```python
from build123d import *

# Parameters (mm, degrees)
SKETCH1_R               = 125
BOSS_EXTRUDE1_DEPTH     = 300
SKETCH2_W               = 100
SKETCH2_H               = 250
CUT_EXTRUDE1_DEPTH      = 200
SKETCH4_R               = 50
CUT_EXTRUDE3_DEPTH      = 60
SKETCH7_R               = 25
CUT_EXTRUDE6_DEPTH      = 176
CUT_EXTRUDE6_DEPTH_BACK = 76
FILLET2_R               = 10
SKETCH8_R               = 45
SKETCH8_R_2             = 25
CUT_EXTRUDE7_DEPTH      = 10
SKETCH10_R              = 45
SKETCH10_R_2            = 25
CUT_EXTRUDE8_DEPTH      = 10


with BuildPart() as part:
    # Sketch1 → Boss-Extrude1 (new body)
    with BuildSketch(Plane(origin=(0, 0, 0), x_dir=(1, 0, 0), z_dir=(0, 1, 0))):
        Circle(SKETCH1_R)
    extrude(amount=BOSS_EXTRUDE1_DEPTH)

    # Sketch2 → Cut-Extrude1 (cut)
    with BuildSketch(Plane(origin=(0, 300, 0), x_dir=(1, 0, 0), z_dir=(0, 1, 0))):
        Rectangle(SKETCH2_W, SKETCH2_H)
    extrude(amount=-CUT_EXTRUDE1_DEPTH, mode=Mode.SUBTRACT)

    # Sketch4 → Cut-Extrude3 (cut)
    with BuildSketch(Plane.XZ):
        Circle(SKETCH4_R)
    extrude(amount=-CUT_EXTRUDE3_DEPTH, mode=Mode.SUBTRACT)

    # Sketch7 → Cut-Extrude6 (cut, two sides)
    with BuildSketch(Plane(origin=(-50, 0, 0), x_dir=(0, 0, -1), z_dir=(1, 0, 0))) as cut_extrude6_sk:
        with BuildLine():
            Line((-87.177978871, 300), (-114.564392374, 300))
            Line((-114.564392374, 300), (-114.564392374, 235))
            ThreePointArc((-114.564392374, 235), (-105.977573518, 269.651471545), (-87.177978871, 300))
        make_face()
        with BuildLine():
            ThreePointArc((87.177978871, 300), (105.977573518, 269.651471545), (114.564392374, 235))
            Line((114.564392374, 235), (114.564392374, 300))
            Line((114.564392374, 300), (87.177978871, 300))
        make_face()
        with Locations((0, 225)):
            Circle(SKETCH7_R)
    extrude(amount=CUT_EXTRUDE6_DEPTH, mode=Mode.SUBTRACT)
    extrude(cut_extrude6_sk.sketch, amount=-CUT_EXTRUDE6_DEPTH_BACK, mode=Mode.SUBTRACT)

    # Fillet2
    fillet2_edges = [part.edges().sort_by_distance(p)[0] for p in [
        (115.807589436, 300, 47.048934409),
        (-125, 300, 0),
    ]]
    fillet(fillet2_edges, radius=FILLET2_R)

    # Sketch8 → Cut-Extrude7 (cut)
    with BuildSketch(Plane(origin=(-125, 0, 0), x_dir=(0, 0, -1), z_dir=(1, 0, 0))):
        with Locations((0, 225)):
            Circle(SKETCH8_R)
        with Locations((0, 225)):
            Circle(SKETCH8_R_2, mode=Mode.SUBTRACT)
    extrude(amount=CUT_EXTRUDE7_DEPTH, mode=Mode.SUBTRACT)

    # Sketch10 → Cut-Extrude8 (cut)
    with BuildSketch(Plane.ZY.offset(-125)):
        with Locations((0, 225)):
            Circle(SKETCH10_R)
        with Locations((0, 225)):
            Circle(SKETCH10_R_2, mode=Mode.SUBTRACT)
    extrude(amount=CUT_EXTRUDE8_DEPTH, mode=Mode.SUBTRACT)


solid = part.part
```
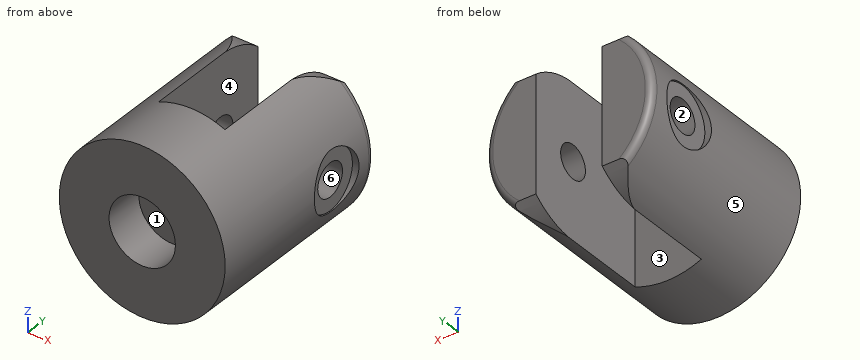
The model under review builds one solid part; all positions refer to its coordinate system, in mm. Face numbers are marked on the shaded views. A direction names the side the tool comes from. Round coordinates to 2 decimals unless told otherwise and drop trailing zeros. Order: outer loops, then holes, each group sorted by start corner. A loop starts at its lowest first (then second) coordinate and runs counter-clockwise, first axis right, second up.
(1) Take a section at C-C, the plane x = 0. State the section outline as (y, z) points.
Working result:
outline: (0, -125) - (100, -125) - (100, 125) - (0, 125) - (0, 50) - (60, 50) - (60, -50) - (0, -50) - close
(2) Tool access review of the marked faces 1, 2 and 3: name each direction out of +Z, -Z, +X, -X, +Y, -Y from which nothing blocks a thin tool from reaching the whole face with its end or side.
Working result:
face 1: -Y
face 2: +X, -X
face 3: +Z, -Z, +Y
(3) For P1, Ø5, axis at y = 58, z = -43.5, coming from the +X side; P2, Ø6, axis at y = 199.5, z = 21.5, coming from the -X side; P3, Ø3, axis at y = 137.5, z = -57, coming from the -X side, all flat-tipped, find the tip position at first contact; note any pin that passes through.
Working result:
P1: stops at x = 118.08
P2: stops at x = -115
P3: stops at x = -112
(4) Mouldability with a two-part tool opening along X and no side actions: class the marked faces 4, 5 and 6 as released by +X, released by -X, zero draft, split by the parting line, or undercut.
Working result:
face 4: undercut
face 5: split by the parting line
face 6: zero draft
(5) Take a section at A-A, the plane z = 0. Count the separate pieces of the cut face and the enclosed holes in it, plus the area to 3 significant figures.
Working result:
separate pieces: 3
enclosed holes: 0
area: 40,700 mm2
(6) Take a section at B-B, the plane y = 225. State the section outline as (x, z) points.
Working result:
outline: (-116.62, -45) arc R125 ccw to (-50, -114.56) - (-50, -25) - (-115, -25) - (-115, -45) - close; (-116.62, 45) - (-115, 45) - (-115, 25) - (-50, 25) - (-50, 114.56) arc R125 ccw to start; (50, -114.56) arc R125 ccw to (116.62, -45) - (115, -45) - (115, -25) - (50, -25) - close; (50, 25) - (115, 25) - (115, 45) - (116.62, 45) arc R125 ccw to (50, 114.56) - close
(7) Take a section at D-D, the plane y = 262.5. State the section outline as (x, z) points.
Working result:
outline: (-122.5, -24.87) arc R125 ccw to (-61.69, -108.71) - (-50, -108.71) - (-50, 108.71) - (-61.69, 108.71) arc R125 ccw to (-122.5, 24.87) - (-115, 24.87) - (-115, -24.87) - close; (50, -108.71) - (61.69, -108.71) arc R125 ccw to (122.5, -24.87) - (115, -24.87) - (115, 24.87) - (122.5, 24.87) arc R125 ccw to (61.69, 108.71) - (50, 108.71) - close
(8) Wall thickness on L1, parallel to Y at x = -116, z = 0; L2, parallel to Y at x = 101, z = 0; L3, parallel to X at y = 263.5, z = 83.5: over which ranges is each line inside the solid? List them lowest first.
Working result:
L1: y = 0 to 180, 270 to 299.95
L2: y = 0 to 200, 250 to 300
L3: x = -93.02 to -50, 50 to 93.02
